Here's how the part is built. I have some questions about the finished solid (model axes, mm). A direction names the side the tool comes from. Coordinates: 2 decimals unless noted, no trailing zeros. Loops run counter-clockwise (first coordinate to the right, second up) from the corner with the lowest first, then second, coordinate; pieces in that order, holes last. Notation, with made-up numbers: (-6.5, 88.5) -> (16.5, 88.5) arc R21 cw to (16.5, 121.5) -> close; hole circle Ø3 at (1.5, 77). An arc over 180 degrees is marked (long way). Answer as a JSON object with one key per item and string values. Group by question number.
Q1. I'm going to push flat-ended pins straight in: pin 1 (4 mm diameter, centred on x = -0.5, y = -17, fed in from -Z); pin 2 (3 mm diameter, centred on x = 4, y = 19, fed in from +Z); pin 3 (5 mm diameter, centred on y = 9.5, z = -6, fed in from +X). Where does each tip first touch, or does it pass through?
Q2. Thinking about a two-plate mould opening in Y: for faces 5 (the conical face through (-5.845, -20.138, 3.356)), 6 (the flat face through (3.2, 22.79, 5.66)), 7 (the conical face through (0.02, 25.36, -6.74)), which applies, released by +Y, released by -Y, zero draft, split by the parting line, or undercut?
Q3. I want a section at A-A on y = -15. Write out the boundary of the cut face in (x, z), then the cut area to 3 significant figures.
Q4. I need wall thicknesses on line 1 (Y direction, x = 0, z = -6); line 2 (Z direction, x = 0.25, y = 2); line 3 (Z direction, x = -1.75, y = -23). Which ranges of each line are inside material? Lowest first, please.
Q5. On a 3-axis mill with a long thin cutter (end or side, diameter ignored), from which of +Z, -Z, +X, -X, +Y, -Y can I reach the whole of each face in a straight line? I mean faces 1 (the conical face through (5.83, 20.14, 3.39)), 2 (the conical face through (-5.83, 20.14, -3.39)), 3 (the conical face through (-5.85, 20.14, 3.36)), 4 (the conical face through (-0.02, -20.14, 6.74)). Say none if no direction works.
```python
from build123d import *

# Parameters (mm, degrees)
SKETCH_2_R          = 12.5
CUT_EXTRUDE_1_DEPTH = 53.92447449


with BuildPart() as part:
    # 草图1 → 旋转1 (revolve)
    with BuildSketch(Plane.XY, mode=Mode.PRIVATE) as revolve_1_sk:
        Polygon((0, 25.5), (10, 25.5), (10, 20), (4, 20), (4, -20), (10, -20), (10, -25.5), (0, -25.5), align=None)
    revolve(revolve_1_sk.sketch.rotate(Axis((0, 0, 0), (0, 1, 0)), 90), axis=Axis((0, 0, 0), (0, 1, 0)))

    # 草图2 → 切除-拉伸1 (cut, through all)
    with BuildSketch(Plane(origin=(0, 25.5, 0), x_dir=(1, 0, 0), z_dir=(0, 1, 0))):
        Circle(SKETCH_2_R)
        Polygon((0, 7.505553499), (-6.5, 3.75277675), (-6.5, -3.75277675), (0, -7.505553499), (6.5, -3.75277675), (6.5, 3.75277675), align=None, mode=Mode.SUBTRACT)
    extrude(amount=-CUT_EXTRUDE_1_DEPTH, mode=Mode.SUBTRACT)

    # 草图3 → 切除-旋转1 (revolve, cut)
    with BuildSketch(Plane.XY):
        Polygon((6.5, 25.5), (9, 25.5), (9, 24.056624327), align=None)
        Polygon((9, 21.443375673), (9, 20), (6.5, 20), align=None)
        Polygon((6.5, -20), (9, -20), (9, -21.443375673), align=None)
        Polygon((6.5, -25.5), (9, -25.5), (9, -24.056624327), align=None)
    revolve(axis=Axis((0, 0, 0), (0, 1, 0)), mode=Mode.SUBTRACT)


solid = part.part
```
Result set:
{
 "1": {"pin 1": "stops at z = -4", "pin 2": "stops at z = 5.84", "pin 3": "stops at x = 1.94"},
 "2": {"face 5": "undercut", "face 6": "zero draft", "face 7": "released by +Y"},
 "3": {"outline": "circle Ø8 at (0, 0)", "area": "50.3 mm²"},
 "4": {"line 1": "y = -25.5 to -20, 20 to 25.5", "line 2": "z = -3.99 to 3.99", "line 3": "z = -6.5 to 6.5"},
 "5": {"face 1": "+Z, +X", "face 2": "-Z, -X", "face 3": "+Z, -X", "face 4": "+Z"}
}
